from build123d import *

# Parameters (mm, degrees)
F0_R     = 79.631708
F6_DEPTH = 86.868
F2_R     = 15.927649
F7_DEPTH = 115.57
F2_R_2   = 15.419675
F8_DEPTH = 116.078
F2_R_3   = 79.631708
F9_DEPTH = 46.736


with BuildPart() as f6:
    # F0 (on Top) → F6 (new body)
    with BuildSketch(Plane.XY):
        Circle(F0_R)
    extrude(amount=F6_DEPTH)

    # F2 (on face) → F7 (join)
    with BuildSketch(Plane.XY):
        with Locations((-29.928552, -38.350657)):
            Circle(F2_R)
    extrude(amount=F7_DEPTH)

    # F2 (on face) → F8 (join)
    with BuildSketch(Plane.XY):
        with Locations((26.319079, -36.545925)):
            Circle(F2_R_2)
    extrude(amount=F8_DEPTH)

    # F2 (on face) → F9 (join)
    with BuildSketch(Plane.XY):
        Circle(F2_R_3)
        with Locations((-29.928552, -38.350657)):
            Circle(F2_R, mode=Mode.SUBTRACT)
        with Locations((26.319079, -36.545925)):
            Circle(F2_R_2, mode=Mode.SUBTRACT)
    extrude(amount=F9_DEPTH)


solid = f6.part
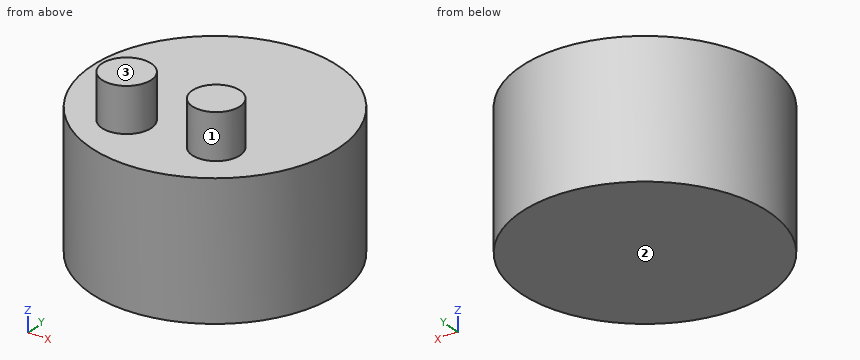
The model under review builds one solid part; all positions refer to its coordinate system, in mm. Face numbers are marked on the shaded views. A direction names the side the tool comes from. Coordinates: 2 decimals unless noted, no trailing zeros. Loops run counter-clockwise (first coordinate to the right, second up) from the corner with the lowest first, then second, coordinate; pieces in that order, holes last. Notation, with made-up numbers: M -33,42 L -25,42 A13 cw -25,46 Z; hole C 21.5,22.5 d9. An arc over 180 degrees is marked long. Put each result on its own line as item: value. Start each with the question number.
Q1. Add section A-A (x = 33.5). Write out the cut boundary in (y, z).
Q2. Clearance check with flat-ended pins moving along their axes: pin 1 (1 mm diameter, centred on x = -35.5, z = 21.5, fed in from -Y); pin 2 (6 mm diameter, centred on y = -22, z = 73, fed in from +X); pin 3 (1 mm diameter, centred on x = 28.5, y = -54, fed in from +Z); pin 4 (10 mm diameter, centred on x = -54, y = 35.5, fed in from -Z). State where each tip first meets the part, or that it passes through.
Q3. Add section D-D (y = 0). Write out the cut boundary in (x, z), and give its area (3 significant figures).
Q4. Add section C-C (z = 79). Write out the cut boundary in (x, y).
Q5. Wall thickness on line 1 (X direction, y = 1, z = 48); line 2 (Z direction, x = -63, y = -17.5); line 3 (X direction, y = -32, z = 89): over which ranges is each line inside the solid? List them lowest first.
Q6. Add section B-B (y = -43). Write out the cut boundary in (x, z).
Q7. For the marked faces 1, 2 and 3, list the 3-axis set-ups (+Z, -Z, +X, -X, +Y, -Y) from which the entire face can be reached by the end or side of a thin tool; tool diameter is ignored.
Answers:
1. outline: M -72.24,0 L 72.24,0 L 72.24,86.87 L -22.9,86.87 L -22.9,116.08 L -50.19,116.08 L -50.19,86.87 L -72.24,86.87 Z
2. pin 1: stops at y = -71.53
2. pin 2: stops at x = 77.33
2. pin 3: stops at z = 86.87
2. pin 4: stops at z = 0
3. outline: M -79.63,0 L 79.63,0 L 79.63,86.87 L -79.63,86.87 Z
3. area: 13,800 mm^2
4. outline: C 0,0 d159.26
5. line 1: x = -79.63 to 79.63
5. line 2: z = 0 to 86.87
5. line 3: x = -44.54 to -15.32, 11.58 to 41.05
6. outline: M -67.02,0 L 67.02,0 L 67.02,86.87 L 40.32,86.87 L 40.32,116.08 L 12.32,116.08 L 12.32,86.87 L -14.69,86.87 L -14.69,115.57 L -45.16,115.57 L -45.16,86.87 L -67.02,86.87 Z
7. face 1: +Z
7. face 2: -Z, +X, -X, +Y, -Y
7. face 3: +Z, -X, +Y, -Y
